Could you check a few things on this drawing? It's one solid part, dimensions in mm from its lowest x, y, z. A direction names the side the tool comes from. Coordinates: 2 decimals unless noted, no trailing zeros. Order: outer loops, then holes, each group sorted by start corner. A loop starts at its lowest first (then second) coordinate and runs counter-clockwise, first axis right, second up. Notation, with made-up numbers: (16, -19.75) - (67, -19.75) arc R28 ccw to (67, 11.25) - close; hole circle Ø3 at (79, 11). An arc over 180 degrees is marked (long way). Answer in a Markdown table with one row per item. Add a question column.
Item 1: If I drill on line 1 along X through (y, z) = (93.25, 7); line 2 along Z through (x, y) = (72.5, 92.75); line 3 along Z through (x, y) = (134, 92.95), over which ranges is the centre line in solid material (lowest first)? Write a range as from..to.
Item 2: I want a section at B-B (x = 134). Please give me the cut outline in (y, z).
Item 3: I want a section at D-D (x = 23). Please give me the cut outline in (y, z).
Item 4: I want a section at A-A (y = 83). Please give me the cut outline in (x, z).
Item 5: I want a section at C-C (z = 7). Please give me the cut outline in (x, y).
Item 6: On a 3-axis mill with a long thin cutter (end or side, diameter ignored), from which of +Z, -Z, +X, -X, +Y, -Y can I reach the whole of each face in a straight line? I mean the marked faces 1, 2 and 3. Say none if no direction works.
Item 7: Will these pins go through, and if not, where does the flat tip stop? pin 1 Ø3 at (x, z) = (88.5, 16.5) entering from -Y; pin 2 Ø11 at (x, z) = (134, 7) entering from +Y; pin 3 Ø3 at (y, z) = (111, 8.5) entering from -X; pin 4 Ø10.5 at (x, y) = (134, 83) entering from +Z.
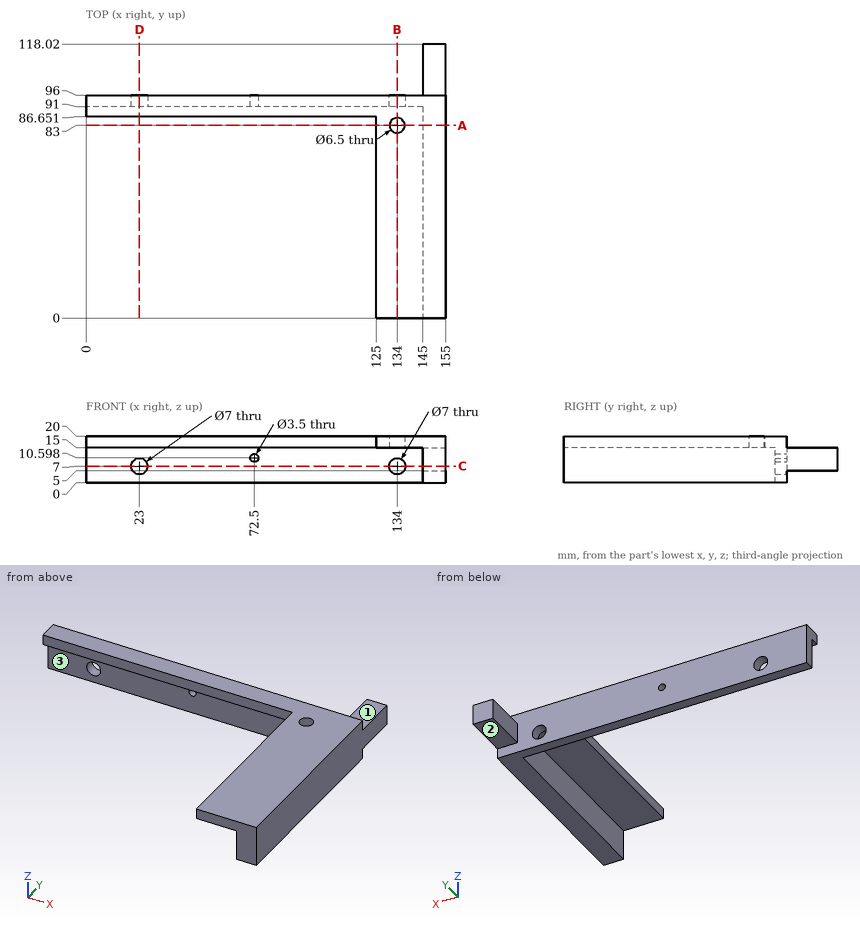
Values follow:
| question | item | result |
|---|---|---|
| 1 | line 1 | x = 0..19.5, 26.5..130.5, 137.5..155 |
| 1 | line 2 | z = 0..8.85, 12.35..20 |
| 1 | line 3 | z = 0..3.5, 10.5..20 |
| 2 | outline | (0, 15) - (79.75, 15) - (79.75, 20) - (0, 20) - close; (86.25, 15) - (91, 15) - (91, 10.5) - (96, 10.5) - (96, 20) - (86.25, 20) - close; (91, 0) - (96, 0) - (96, 3.5) - (91, 3.5) - close |
| 3 | outline | (86.65, 15) - (91, 15) - (91, 10.5) - (96, 10.5) - (96, 20) - (86.65, 20) - close; (91, 0) - (96, 0) - (96, 3.5) - (91, 3.5) - close |
| 4 | outline | (125, 15) - (130.75, 15) - (130.75, 20) - (125, 20) - close; (137.25, 15) - (145, 15) - (145, 0) - (155, 0) - (155, 20) - (137.25, 20) - close |
| 5 | outline | (0, 91) - (19.5, 91) - (19.5, 96) - (0, 96) - close; (26.5, 91) - (130.5, 91) - (130.5, 96) - (26.5, 96) - close; (137.5, 91) - (145, 91) - (145, 0) - (155, 0) - (155, 118.02) - (145, 118.02) - (145, 96) - (137.5, 96) - close |
| 6 | face 1 | +Z, +X, -X, +Y |
| 6 | face 2 | -Z, +X, -X, +Y |
| 6 | face 3 | -Z, -X, -Y |
| 7 | pin 1 | stops at y = 86.65 |
| 7 | pin 2 | stops at y = 96 |
| 7 | pin 3 | stops at x = 145 |
| 7 | pin 4 | stops at z = 20 |
